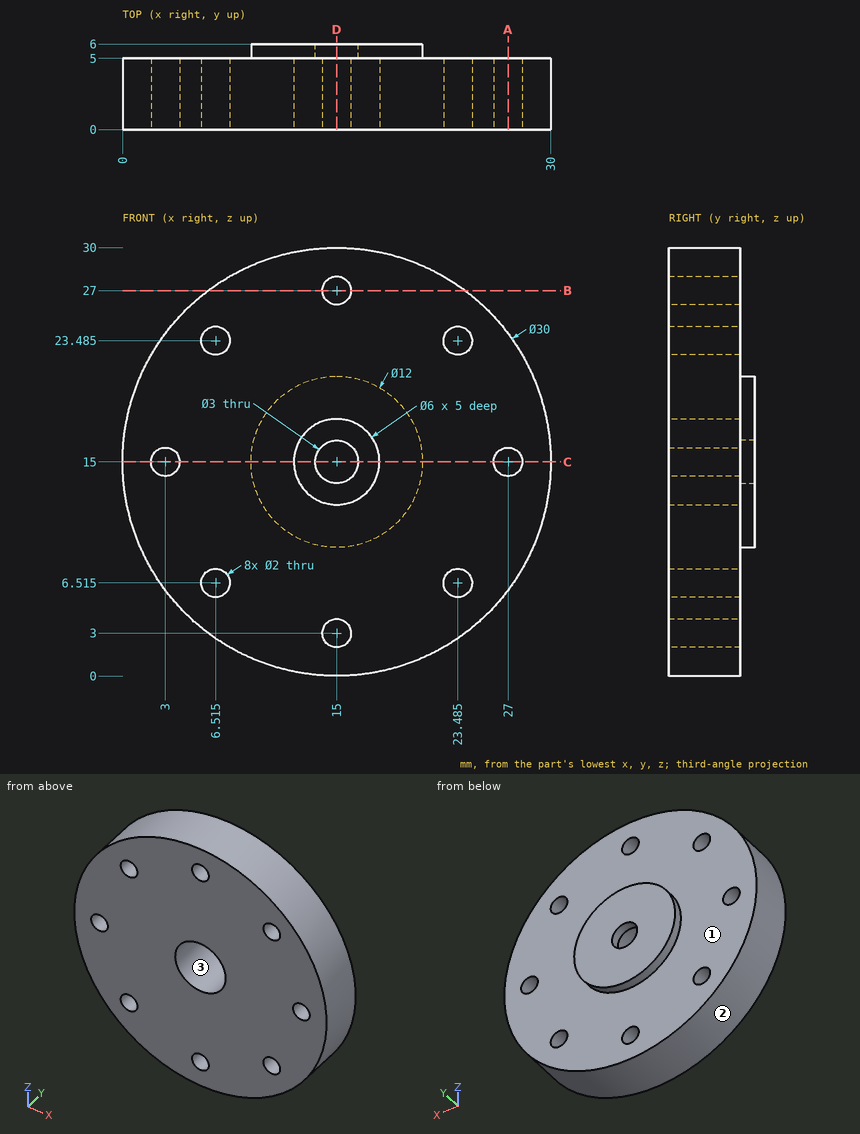
Geometry check sheet. Reference: drawing and pictorial views, mm from the part's lowest x, y, z. Round coordinates to 2 decimals unless told otherwise and drop trailing zeros. Order: outer loops, then holes, each group sorted by start corner. A loop starts at its lowest first (then second) coordinate and runs counter-clockwise, first axis right, second up. Notation, with made-up numbers: M 88.25,-39 L 122.25,-39 A30 cw 122.25,-11 Z; hole C 26.25,52.25 d6. An arc over 180 degrees is marked long. Write item = value, one per line.
Q1. Section check A-A (x = 27). Enter the section's corners in (y, z), plus the area to 3 significant figures.
Answer block:
outline = M 0,6 L 5,6 L 5,14 L 0,14 Z; M 0,16 L 5,16 L 5,24 L 0,24 Z
area = 80.0 mm^2
Q2. Section check C-C (z = 15). Enter the section's corners in (x, y).
Answer block:
outline = M 0,0 L 2,0 L 2,5 L 0,5 Z; M 4,0 L 12,0 L 12,5 L 13.5,5 L 13.5,6 L 9,6 L 9,5 L 4,5 Z; M 16.5,5 L 18,5 L 18,0 L 26,0 L 26,5 L 21,5 L 21,6 L 16.5,6 Z; M 28,0 L 30,0 L 30,5 L 28,5 Z
Q3. Depth check by flat-ended pin: pin 1 Ø3 at (x, z) = (23.49, 6.51) entering from +Y; pin 2 Ø1.8 at (x, z) = (23.49, 23.49) entering from -Y; pin 3 Ø2 at (y, z) = (1.5, 21) entering from +X; pin 4 Ø4 at (x, z) = (15, 15) entering from -Y. Enter the tip coordinate at first touch or a pass-through.
Answer block:
pin_1 = 5
pin_2 = through
pin_3 = 29.14
pin_4 = 5
Q4. Scan lines: line 1 (X direction, y = 2.8, z = 15); line 2 (Z direction, x = 23, y = 0.4); line 3 (Z direction, x = 23.25, y = 1.55). Record each from-to range of solid material in increasing order.
Answer block:
line_1 = 0 to 2, 4 to 12, 18 to 26, 28 to 30
line_2 = 2.31 to 5.64, 7.39 to 22.61, 24.36 to 27.69
line_3 = 2.47 to 5.54, 7.49 to 22.51, 24.46 to 27.53
Q5. Section check B-B (z = 27). Enter the section's corners in (x, y).
Answer block:
outline = M 6,0 L 14,0 L 14,5 L 6,5 Z; M 16,0 L 24,0 L 24,5 L 16,5 Z
Q6. Section check D-D (x = 15). Enter the section's corners in (y, z), plus the area to 3 significant figures.
Answer block:
outline = M 0,0 L 5,0 L 5,2 L 0,2 Z; M 0,4 L 5,4 L 5,9 L 6,9 L 6,13.5 L 5,13.5 L 5,12 L 0,12 Z; M 0,18 L 5,18 L 5,16.5 L 6,16.5 L 6,21 L 5,21 L 5,26 L 0,26 Z; M 0,28 L 5,28 L 5,30 L 0,30 Z
area = 109 mm^2
Q7. Release check for a two-part mould opening along Z. For the marked faces 1, 2 and 3 record: released by +Z, released by -Z, zero draft, split by the parting line, or undercut.
Answer block:
face_1 = zero draft
face_2 = split by the parting line
face_3 = undercut
